Study the drawing (mm; zero at the part's minimum x, y, z) and answer. Round coordinates to 2 decimals unless told otherwise and drop trailing zeros. Loops run counter-clockwise (first coordinate to the right, second up) from the corner with the lowest first, then second, coordinate; pieces in that order, holes last. Notation, with made-up numbers: M -13,40 L 24,40 A8 cw 24,45 Z; hole C 48.25,87 d3. An arc over 180 degrees is marked long. Put each result on its own line as item: value. Start each with the question number.
(1) Section B-B, the plane y = 37 is taken. Determine the outline of the cut face in (x, z).
(2) Determine the mould class of the marked faces 1, 2, 3 and 4 for opening direction Y: released by +Y, released by -Y, zero draft, split by the parting line, or undercut.
(3) Section D-D, the plane x = 3.5 is taken. Determine the outline of the cut face in (y, z).
(4) Section A-A, the plane x = 25.4 is taken. Determine the outline of the cut face in (y, z).
(5) Straight lines are drawn through the part: line 1 (Y direction, x = 25.4, z = 1.75); line 2 (X direction, y = 30, z = 4.25) (1 decimal); line 3 (X direction, y = 18.5, z = 5.5). For each, find the intervals that lie inside material, in ascending order.
(6) A flat-ended cylindrical pin translates along its axis: P1, Ø1, axis at y = 12, z = 2.5, coming from the -X side. Find the tip coordinate at first contact, or state that the pin passes through.
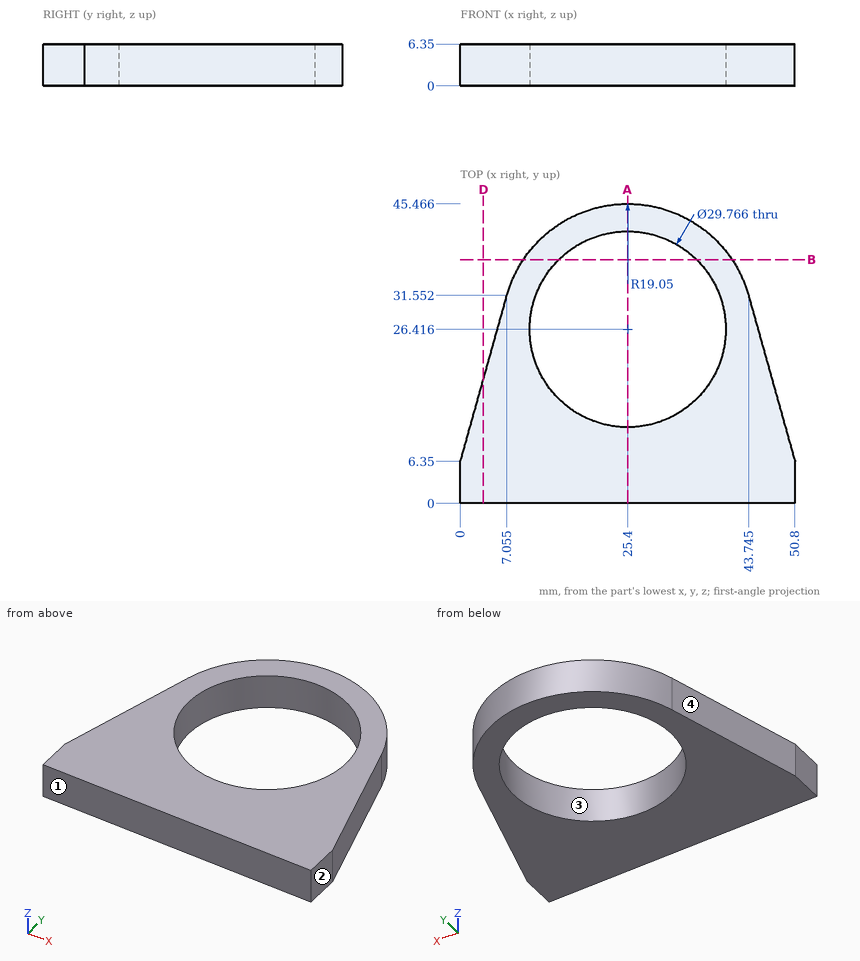
Recorded:
1. outline: M 9.56,0 L 14.94,0 L 14.94,6.35 L 9.56,6.35 Z; M 35.86,0 L 41.24,0 L 41.24,6.35 L 35.86,6.35 Z
2. face 1: released by -Y
2. face 2: zero draft
2. face 3: undercut
2. face 4: released by +Y
3. outline: M 0,0 L 18.85,0 L 18.85,6.35 L 0,6.35 Z
4. outline: M 0,0 L 11.53,0 L 11.53,6.35 L 0,6.35 Z; M 41.3,0 L 45.47,0 L 45.47,6.35 L 41.3,6.35 Z
5. line 1: y = 0 to 11.53, 41.3 to 45.47
5. line 2: x = 6.6 to 11, 39.8 to 44.2
5. line 3: x = 3.4 to 12.8, 38 to 47.4
6. P1: stops at x = 1.44
